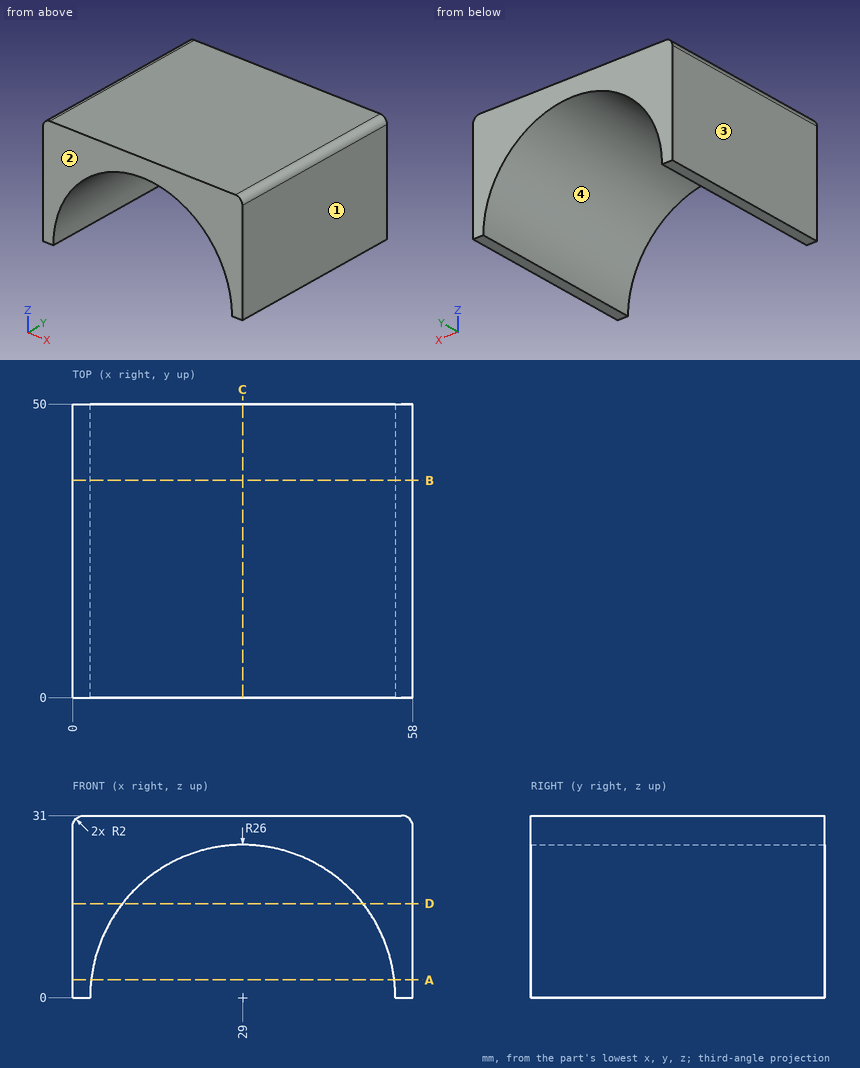
The drawing under review shows one solid part. Ordinate dimensions are in mm from its lowest x, y, z. Coordinates: 2 decimals unless noted, no trailing zeros. Order: outer loops, then holes, each group sorted by start corner. A loop starts at its lowest first (then second) coordinate and runs counter-clockwise, first axis right, second up. Notation, with made-up numbers: M 86.5,44.5 L 102.5,44.5 A7 cw 102.5,55.5 Z; hole C 75,-18.75 d1. An arc over 180 degrees is marked long. One line per question, with ' | ' between items.
(1) Add section B-B, the plane y = 37. Write out the cut boundary in (x, z).
Geometry results:
outline: M 0,0 L 3,0 A26 cw 55,0 L 58,0 L 58,29 A2 ccw 56,31 L 2,31 A2 ccw 0,29 Z
(2) Add section A-A, the plane z = 3. Write out the cut boundary in (x, y), then the cut area to 3 significant figures.
Geometry results:
outline: M 0,0 L 3.17,0 L 3.17,50 L 0,50 Z; M 54.83,0 L 58,0 L 58,50 L 54.83,50 Z | area: 317 mm²
(3) The part is to be moulded in two halves that separate along X. For the marked faces 1, 2, 3 and 4, say which applies: +X half, -X half, draft (parallel to the pull), parting line (faces both ways), or undercut.
Geometry results:
face 1: +X half | face 2: draft | face 3: -X half | face 4: undercut
(4) Add section D-D, the plane z = 16. Write out the cut boundary in (x, y).
Geometry results:
outline: M 0,0 L 8.51,0 L 8.51,50 L 0,50 Z; M 49.49,0 L 58,0 L 58,50 L 49.49,50 Z
(5) For probe 1 along X at (y, z) = (40.5, 4); probe 2 along X at (y, z) = (30.5, 18); probe 3 along Z at (x, y) = (49.5, 38), list the stretches that pass through material, from the lowest coordinate up. Write a range as from..to.
Geometry results:
probe 1: x = 0..3.31, 54.69..58 | probe 2: x = 0..10.24, 47.76..58 | probe 3: z = 15.99..31
(6) Insertion check: pin 1 (1 mm diameter, centred on y = 9, z = 21, fed in from -X); pin 2 (10 mm diameter, centred on x = 18, y = 33, fed in from -Z); pin 3 (10 mm diameter, centred on x = 48.5, z = 4.5, fed in from -Y); pin 4 (6 mm diameter, centred on x = 9, y = 27, fed in from -Z). Each pin has a flat end and moves straight along its axis. Give the tip position at first contact, or say it passes through.
Geometry results:
pin 1: stops at x = 0 | pin 2: stops at z = 20.49 | pin 3: passes through | pin 4: stops at z = 12.12
(7) Add section C-C, the plane x = 29. Write out the cut boundary in (y, z).
Geometry results:
outline: M 0,26 L 50,26 L 50,31 L 0,31 Z
